Read the model definition and answer for the solid it produces. Units are mm, in the model's axes. A direction names the side the tool comes from. Round coordinates to 2 decimals unless told otherwise and drop trailing zeros. Order: outer loops, then holes, each group sorted by start corner. A loop starts at its lowest first (then second) coordinate and runs counter-clockwise, first axis right, second up. Notation, with made-up numbers: M 10.5,15 L 60.5,15 A28 cw 60.5,41 Z; hole C 3,-24.5 d11. An arc over 180 degrees is marked long. Use one line per item in the form item = value. Start each with the question number.
from build123d import *

# Parameters (mm, degrees)
F0_W     = 127
F0_H     = 127
F1_DEPTH = 152.4
F2_R     = 50.8
F3_DEPTH = 127
F4_W     = 101.6
F4_H     = 119.7034602863
F5_DEPTH = 63.5
F6_R     = 6.35
F7_DEPTH = 127


with BuildPart() as f1:
    # F0 (on Top) → F1 (new body)
    with BuildSketch(Plane.XY):
        Rectangle(F0_W, F0_H)
    extrude(amount=F1_DEPTH)

    # F2 (on face) → F3 (cut)
    with BuildSketch(Plane.XY.offset(152.4)):
        Circle(F2_R)
    extrude(amount=-F3_DEPTH, mode=Mode.SUBTRACT)

    # F4 (on Front) → F5 (cut, symmetric)
    with BuildSketch(Plane.XZ):
        with Locations((0, -9.0517301432)):
            Rectangle(F4_W, F4_H)
    extrude(amount=F5_DEPTH, both=True, mode=Mode.SUBTRACT)

    # F6 (on face) → F7 (cut)
    with BuildSketch(Plane.YZ.offset(63.5)):
        with Locations((0, 12.7)):
            Circle(F6_R)
    extrude(amount=-F7_DEPTH, mode=Mode.SUBTRACT)


solid = f1.part
Item 1: Section A-A (z = 12.7) is taken. Write down the section's boundary in (x, y), and give its area (3 significant figures).
Item 2: Section C-C (y = 55.5) is taken. Write down the section's boundary in (x, z).
Item 3: For a pull along Y with two mould halves and no side action, classify faces 1 (the flat face through (-1, 63.5, 92)), 2 (the cylindrical face through (-11.012, -49.592, 102.311)), 3 (the flat face through (-43, 29, 152.4)), 4 (the flat face through (-1, -63.5, 92)) as pulls with the +Y half, pulls with the -Y half, needs draft (parallel to the pull), parting line crosses it, or undercut.
Item 4: Find the intervals of material crossed by L1, parallel to X at y = -10.5, z = 50; L2, parallel to Z at x = 60, y = 0, in increasing order. Write a range as [from, to].
Item 5: Given P1, Ø4, axis at x = -48.5, y = 40.5, coming from the -Z side, flat-ended and moving along its own axis, determine where the tip first touches the part or whether it passes through.
Item 6: Section D-D (x = -18) is taken. Write down the section's boundary in (y, z).
Item 7: Section B-B (z = 32.5) is taken. Write down the section's boundary in (x, y), and give its area (3 significant figures).
Item 8: A tool of negligible diameter and unlimited length cuts with its end or side. For faces 5 (the cylindrical face through (57.239, 3.414, 18.054)), 6 (the flat face through (-1, -53, 50.8)), from which of +Z, -Z, +X, -X, +Y, -Y can it reach the whole face along a straight path? Write none if from no direction.
The answers:
q1.outline = M -63.5,-63.5 L -50.8,-63.5 L -50.8,-6.35 L -63.5,-6.35 Z; M -63.5,6.35 L -50.8,6.35 L -50.8,63.5 L -63.5,63.5 Z; M 50.8,-63.5 L 63.5,-63.5 L 63.5,-6.35 L 50.8,-6.35 Z; M 50.8,6.35 L 63.5,6.35 L 63.5,63.5 L 50.8,63.5 Z
q1.area = 2,900 mm²
q2.outline = M -63.5,0 L -50.8,0 L -50.8,50.8 L 50.8,50.8 L 50.8,0 L 63.5,0 L 63.5,152.4 L -63.5,152.4 Z
q3.face_1 = pulls with the +Y half
q3.face_2 = undercut
q3.face_3 = needs draft
q3.face_4 = pulls with the -Y half
q4.L1 = [-63.5, -50.8], [50.8, 63.5]
q4.L2 = [0, 6.35], [19.05, 152.4]
q5.P1 = 50.8
q6.outline = M -63.5,50.8 L -47.5,50.8 L -47.5,152.4 L -63.5,152.4 Z; M 47.5,50.8 L 63.5,50.8 L 63.5,152.4 L 47.5,152.4 Z
q7.outline = M -63.5,-63.5 L -50.8,-63.5 L -50.8,63.5 L -63.5,63.5 Z; M 50.8,-63.5 L 63.5,-63.5 L 63.5,63.5 L 50.8,63.5 Z
q7.area = 3,230 mm²
q8.face_5 = +X, -X
q8.face_6 = -Z, +Y, -Y
